```python
from build123d import *

# Parameters (mm, degrees)
F0_W     = 100
F0_H     = 100
F0_W_2   = 15
F0_H_2   = 15
F0_R     = 4.7625
F0_R_2   = 3.55
F0_W_3   = 64
F0_H_3   = 38
F1_DEPTH = 15
F2_DEPTH = 80
F0_R_3   = 2.05
F3_DEPTH = 76.6
F4_DEPTH = 7
F5_DEPTH = 11.6
F6_DEPTH = 35
F7_START = 4.2
F7_DEPTH = 30.8
F8_START = 4.2
F8_DEPTH = 10.8
F9_DEPTH = 60


with BuildPart() as f1:
    # F0 (on Top) → F1 (new body)
    with BuildSketch(Plane.XY):
        with Locations((-0.0015218393, -0.0144693477)):
            Rectangle(F0_W, F0_H)
        with Locations((-40.0015218393, -40.0144693477)):
            Rectangle(F0_W_2, F0_H_2, mode=Mode.SUBTRACT)
        with Locations((-24.5015218393, -24.5144693477)):
            Circle(F0_R, mode=Mode.SUBTRACT)
        Polygon((4.097665072, -40.0144693477), (2.0480716163, -43.5644693477), (-2.0511152949, -43.5644693477), (-4.1007087505, -40.0144693477), (-2.0511152949, -36.4644693477), (2.0480716163, -36.4644693477), align=None, mode=Mode.SUBTRACT)
        with Locations((39.9984781607, -40.0144693477)):
            Rectangle(F0_W_2, F0_H_2, mode=Mode.SUBTRACT)
        with Locations((-0.0015218393, -24.5144693477)):
            Circle(F0_R_2, mode=Mode.SUBTRACT)
        with Locations((24.4984781607, -24.5144693477)):
            Circle(F0_R, mode=Mode.SUBTRACT)
        Polygon((-35.902334928, -0.0144693477), (-37.9519283837, -3.5644693477), (-42.0511152949, -3.5644693477), (-44.1007087505, -0.0144693477), (-42.0511152949, 3.5355306523), (-37.9519283837, 3.5355306523), align=None, mode=Mode.SUBTRACT)
        with Locations((-24.5015218393, 24.4855306523)):
            Circle(F0_R, mode=Mode.SUBTRACT)
        with Locations((-40.0015218393, 39.9855306523)):
            Rectangle(F0_W_2, F0_H_2, mode=Mode.SUBTRACT)
        Polygon((4.097665072, 39.9855306523), (2.0480716163, 36.4355306523), (-2.0511152949, 36.4355306523), (-4.1007087505, 39.9855306523), (-2.0511152949, 43.5355306523), (2.0480716163, 43.5355306523), align=None, mode=Mode.SUBTRACT)
        with Locations((-0.0015218393, -0.0144693477)):
            Rectangle(F0_W_3, F0_H_3, mode=Mode.SUBTRACT)
        with Locations((-0.0015218393, 24.4855306523)):
            Circle(F0_R_2, mode=Mode.SUBTRACT)
        with Locations((24.4984781607, 24.4855306523)):
            Circle(F0_R, mode=Mode.SUBTRACT)
        Polygon((42.0480716163, -3.5644693477), (37.9488847051, -3.5644693477), (35.8992912495, -0.0144693477), (37.9488847051, 3.5355306523), (42.0480716163, 3.5355306523), (44.097665072, -0.0144693477), align=None, mode=Mode.SUBTRACT)
        with Locations((39.9984781607, 39.9855306523)):
            Rectangle(F0_W_2, F0_H_2, mode=Mode.SUBTRACT)
    extrude(amount=F1_DEPTH)

    # F0 (on Top) → F2 (join)
    with BuildSketch(Plane.XY):
        with Locations((-40.0015218393, -40.0144693477)):
            Rectangle(F0_W_2, F0_H_2)
        Polygon((-35.902334928, -40.0144693477), (-37.9519283837, -43.5644693477), (-42.0511152949, -43.5644693477), (-44.1007087505, -40.0144693477), (-42.0511152949, -36.4644693477), (-37.9519283837, -36.4644693477), align=None, mode=Mode.SUBTRACT)
        with Locations((39.9984781607, -40.0144693477)):
            Rectangle(F0_W_2, F0_H_2)
        Polygon((44.097665072, -40.0144693477), (42.0480716163, -43.5644693477), (37.9488847051, -43.5644693477), (35.8992912495, -40.0144693477), (37.9488847051, -36.4644693477), (42.0480716163, -36.4644693477), align=None, mode=Mode.SUBTRACT)
        with Locations((-40.0015218393, 39.9855306523)):
            Rectangle(F0_W_2, F0_H_2)
        Polygon((-42.0511152949, 43.5355306523), (-37.9519283837, 43.5355306523), (-35.902334928, 39.9855306523), (-37.9519283837, 36.4355306523), (-42.0511152949, 36.4355306523), (-44.1007087505, 39.9855306523), align=None, mode=Mode.SUBTRACT)
        with Locations((39.9984781607, 39.9855306523)):
            Rectangle(F0_W_2, F0_H_2)
        Polygon((42.0480716163, 36.4355306523), (37.9488847051, 36.4355306523), (35.8992912495, 39.9855306523), (37.9488847051, 43.5355306523), (42.0480716163, 43.5355306523), (44.097665072, 39.9855306523), align=None, mode=Mode.SUBTRACT)
    extrude(amount=F2_DEPTH)

    # F0 (on Top) → F3 (join)
    with BuildSketch(Plane.XY):
        Polygon((-35.902334928, 39.9855306523), (-37.9519283837, 43.5355306523), (-42.0511152949, 43.5355306523), (-44.1007087505, 39.9855306523), (-42.0511152949, 36.4355306523), (-37.9519283837, 36.4355306523), align=None)
        with Locations((-40.0015218393, 39.9855306523)):
            Circle(F0_R_3, mode=Mode.SUBTRACT)
        Polygon((35.8992912495, 39.9855306523), (37.9488847051, 36.4355306523), (42.0480716163, 36.4355306523), (44.097665072, 39.9855306523), (42.0480716163, 43.5355306523), (37.9488847051, 43.5355306523), align=None)
        with Locations((39.9984781607, 39.9855306523)):
            Circle(F0_R_3, mode=Mode.SUBTRACT)
        Polygon((37.9488847051, -43.5644693477), (42.0480716163, -43.5644693477), (44.097665072, -40.0144693477), (42.0480716163, -36.4644693477), (37.9488847051, -36.4644693477), (35.8992912495, -40.0144693477), align=None)
        with Locations((39.9984781607, -40.0144693477)):
            Circle(F0_R_3, mode=Mode.SUBTRACT)
        Polygon((-42.0511152949, -43.5644693477), (-37.9519283837, -43.5644693477), (-35.902334928, -40.0144693477), (-37.9519283837, -36.4644693477), (-42.0511152949, -36.4644693477), (-44.1007087505, -40.0144693477), align=None)
        with Locations((-40.0015218393, -40.0144693477)):
            Circle(F0_R_3, mode=Mode.SUBTRACT)
    extrude(amount=F3_DEPTH)

    # F0 (on Top) → F4 (join)
    with BuildSketch(Plane.XY):
        with Locations((-0.0015218393, -0.0144693477)):
            Rectangle(F0_W_3, F0_H_3)
    extrude(amount=F4_DEPTH)

    # F0 (on Top) → F5 (join)
    with BuildSketch(Plane.XY):
        Polygon((-42.0511152949, -3.5644693477), (-37.9519283837, -3.5644693477), (-35.902334928, -0.0144693477), (-37.9519283837, 3.5355306523), (-42.0511152949, 3.5355306523), (-44.1007087505, -0.0144693477), align=None)
        with Locations((-40.0015218393, -0.0144693477)):
            Circle(F0_R_3, mode=Mode.SUBTRACT)
        Polygon((-2.0511152949, -43.5644693477), (2.0480716163, -43.5644693477), (4.097665072, -40.0144693477), (2.0480716163, -36.4644693477), (-2.0511152949, -36.4644693477), (-4.1007087505, -40.0144693477), align=None)
        with Locations((-0.0015218393, -40.0144693477)):
            Circle(F0_R_3, mode=Mode.SUBTRACT)
        Polygon((35.8992912495, -0.0144693477), (37.9488847051, -3.5644693477), (42.0480716163, -3.5644693477), (44.097665072, -0.0144693477), (42.0480716163, 3.5355306523), (37.9488847051, 3.5355306523), align=None)
        with Locations((39.9984781607, -0.0144693477)):
            Circle(F0_R_3, mode=Mode.SUBTRACT)
        Polygon((-2.0511152949, 36.4355306523), (2.0480716163, 36.4355306523), (4.097665072, 39.9855306523), (2.0480716163, 43.5355306523), (-2.0511152949, 43.5355306523), (-4.1007087505, 39.9855306523), align=None)
        with Locations((-0.0015218393, 39.9855306523)):
            Circle(F0_R_3, mode=Mode.SUBTRACT)
    extrude(amount=F5_DEPTH)

    # F0 (on Top) → F6 (join)
    with BuildSketch(Plane.XY):
        with Locations((-24.5015218393, 24.4855306523)):
            Circle(F0_R)
        with Locations((-24.5015218393, 24.4855306523)):
            Circle(F0_R_2, mode=Mode.SUBTRACT)
        with Locations((24.4984781607, 24.4855306523)):
            Circle(F0_R)
        with Locations((24.4984781607, 24.4855306523)):
            Circle(F0_R_2, mode=Mode.SUBTRACT)
        with Locations((24.4984781607, -24.5144693477)):
            Circle(F0_R)
        with Locations((24.4984781607, -24.5144693477)):
            Circle(F0_R_2, mode=Mode.SUBTRACT)
        with Locations((-24.5015218393, -24.5144693477)):
            Circle(F0_R)
        with Locations((-24.5015218393, -24.5144693477)):
            Circle(F0_R_2, mode=Mode.SUBTRACT)
    extrude(amount=F6_DEPTH)

    # F0 (on Top) → F7 (join)
    with BuildSketch(Plane.XY.offset(F7_START)):
        with Locations((-24.5015218393, 24.4855306523)):
            Circle(F0_R_2)
        with Locations((-24.5015218393, 24.4855306523)):
            Circle(F0_R_3, mode=Mode.SUBTRACT)
        with Locations((24.4984781607, 24.4855306523)):
            Circle(F0_R_2)
        with Locations((24.4984781607, 24.4855306523)):
            Circle(F0_R_3, mode=Mode.SUBTRACT)
        with Locations((24.4984781607, -24.5144693477)):
            Circle(F0_R_2)
        with Locations((24.4984781607, -24.5144693477)):
            Circle(F0_R_3, mode=Mode.SUBTRACT)
        with Locations((-24.5015218393, -24.5144693477)):
            Circle(F0_R_2)
        with Locations((-24.5015218393, -24.5144693477)):
            Circle(F0_R_3, mode=Mode.SUBTRACT)
    extrude(amount=F7_DEPTH)

    # F0 (on Top) → F8 (join)
    with BuildSketch(Plane.XY.offset(F8_START)):
        with Locations((-0.0015218393, -24.5144693477)):
            Circle(F0_R_2)
        with Locations((-0.0015218393, -24.5144693477)):
            Circle(F0_R_3, mode=Mode.SUBTRACT)
        with Locations((-0.0015218393, 24.4855306523)):
            Circle(F0_R_2)
        with Locations((-0.0015218393, 24.4855306523)):
            Circle(F0_R_3, mode=Mode.SUBTRACT)
    extrude(amount=F8_DEPTH)

    # F0 (on Top) → F9 (join)
    with BuildSketch(Plane.XY):
        with Locations((-40.0015218393, 39.9855306523)):
            Circle(F0_R_3)
        with Locations((39.9984781607, 39.9855306523)):
            Circle(F0_R_3)
        with Locations((39.9984781607, -40.0144693477)):
            Circle(F0_R_3)
        with Locations((-40.0015218393, -40.0144693477)):
            Circle(F0_R_3)
    extrude(amount=F9_DEPTH)


solid = f1.part
```
Geometry: final body of the model. Coordinates: model frame, mm. A direction names the side the tool comes from. Coordinates: 2 decimals unless noted, no trailing zeros. Order: outer loops, then holes, each group sorted by start corner. A loop starts at its lowest first (then second) coordinate and runs counter-clockwise, first axis right, second up. Notation, with made-up numbers: (73, 0.25) - (125, 0.25) arc R16 cw to (125, 22.25) - close; hole circle Ø10 at (-9, 31.25). An arc over 180 degrees is marked (long way). Return JSON: item names as keys, results as strings. Group by question number.
1. Cut plane A-A (z = 57.5). Output: boundary loops of the cut face in (x, y), plus the area to 3 significant figures.
2. Material intervals for line 1 along Y through (x, z) = (34.5, 24); line 2 along X through (y, z) = (-35, 66); line 3 along Y through (x, z) = (7, 13), sorted ascending. Write a range as [from, to].
3. Pull-direction query (Y, two-part tool) for faces 6 (the face through (-47.502, 40, 47)), 7 (the face through (-40, -47.514, 47)), 8 (the face through (-36.91, 38.24, 78.28)), 9 (the face through (42, 2, 11.6)); classes: pulls with the +Y half, pulls with the -Y half, needs draft (parallel to the pull), parting line crosses it, or undercut.
4. Cut plane C-C (y = 11). Output: boundary loops of the cut face in (x, z), plus the area to 3 significant figures.
5. Cut plane B-B (z = 33.5). Count the separate pieces of the cut face and the enclosed holes in it, plus the area to 3 significant figures.
6. Set-up query: faces 1 (the face through (-1, 1, 0)), 2 (the face through (40, -47.514, 47)), 3 (the face through (-40, 47.486, 47)), 4 (the face through (40, 32.486, 47)), 5 (the face through (-40, 40, 60)). Return all of +Z, -Z, +X, -X, +Y, -Y with unobstructed straight access to the full face (end or side cutting, diameter ignored); none if empty.
7. Pin query (flat end, axial travel): pin 1 (3.5 mm diameter, centred on x = 0, y = 24.49, fed in from -Z); pin 2 (1.7 mm diameter, centred on x = 40, z = 79, fed in from -Y); pin 3 (10 mm diameter, centred on y = 32.5, z = 42, fed in from -X); pin 4 (6 mm diameter, centred on x = -16.5, y = 16.5, fed in from +Z). Return the tip coordinate at first contact, or that it passes through.
Resolved:
{
 "1": {"outline": "(-47.5, -47.51) - (-32.5, -47.51) - (-32.5, -32.51) - (-47.5, -32.51) - close; (-47.5, 32.49) - (-32.5, 32.49) - (-32.5, 47.49) - (-47.5, 47.49) - close; (32.5, -47.51) - (47.5, -47.51) - (47.5, -32.51) - (32.5, -32.51) - close; (32.5, 32.49) - (47.5, 32.49) - (47.5, 47.49) - (32.5, 47.49) - close", "area": "900 mm²"},
 "2": {"line 1": "y = [-47.51, -32.51], [32.49, 47.49]", "line 2": "x = [-47.5, -32.5], [32.5, 47.5]", "line 3": "y = [-50.01, -19.01], [18.99, 49.99]"},
 "3": {"face 6": "needs draft", "face 7": "pulls with the -Y half", "face 8": "undercut", "face 9": "undercut"},
 "4": {"outline": "(-50, 0) - (50, 0) - (50, 15) - (32, 15) - (32, 7) - (-32, 7) - (-32, 15) - (-50, 15) - close", "area": "988 mm²"},
 "5": {"separate pieces": "8", "enclosed holes": "4", "area": "1,130 mm²"},
 "6": {"face 1": "-Z, +X, -X, +Y, -Y", "face 2": "+Z, +X, -X, -Y", "face 3": "+Z, +X, -X, +Y", "face 4": "+Z, +X, -X", "face 5": "+Z"},
 "7": {"pin 1": "passes through", "pin 2": "stops at y = -47.51", "pin 3": "stops at x = -47.5", "pin 4": "stops at z = 15"}
}
